For this review, use the dimensioned drawing (mm, ordinates from the lowest corner) and the shaded views. A direction names the side the tool comes from. Give positions to 0.01 mm unless a question says otherwise; leave off trailing zeros. Write each loop counter-clockwise with the first axis right and the second up, starting at its lowest first coordinate (ties: lowest second). Pieces come first, ordered by that corner, then holes. Notation, with made-up numbers: (-13.5, -20) -> (36.5, -20) arc R13 ccw to (36.5, -13) -> close; hole circle Ø3 at (-10.75, 21). An arc over 180 degrees is marked (long way). Answer as CSV lines item,"result".
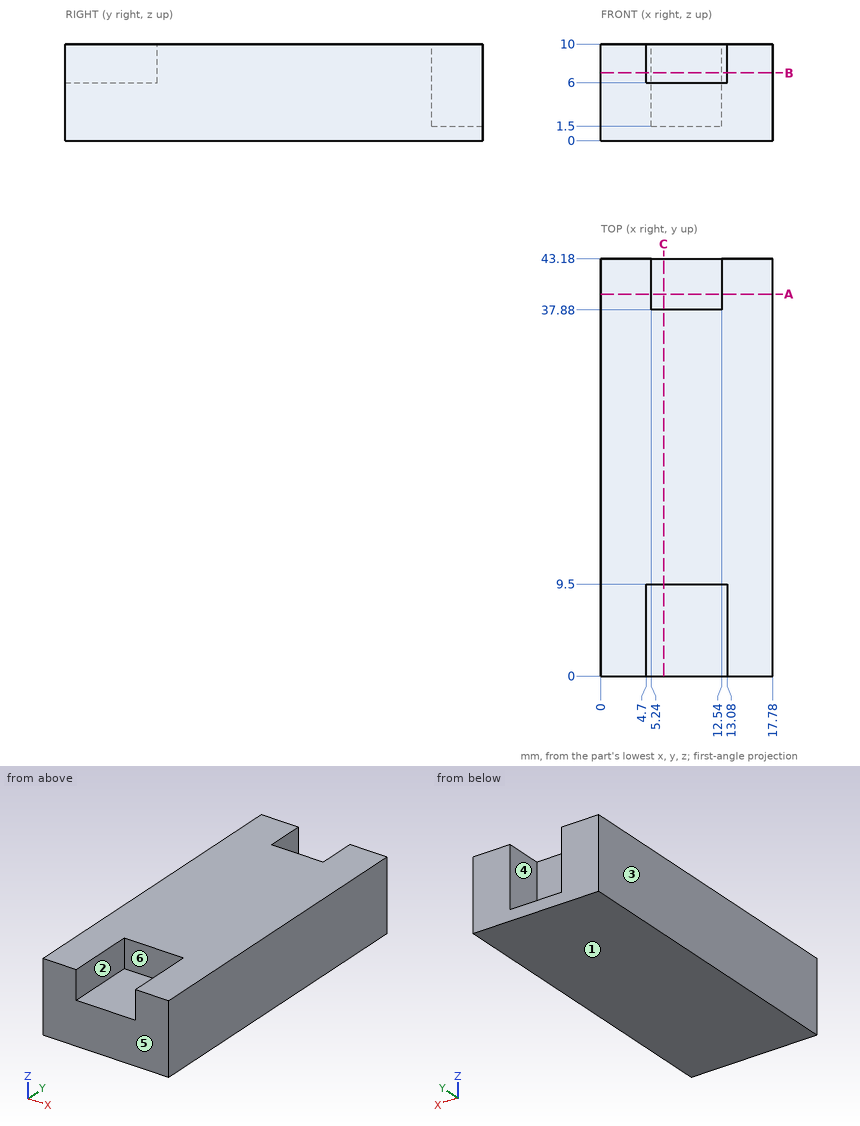
Q1. Add section B-B (z = 7). Write out the cut boundary in (x, y).
Answer block:
outline,"(0, 0) -> (4.7, 0) -> (4.7, 9.5) -> (13.08, 9.5) -> (13.08, 0) -> (17.78, 0) -> (17.78, 43.18) -> (12.54, 43.18) -> (12.54, 37.88) -> (5.24, 37.88) -> (5.24, 43.18) -> (0, 43.18) -> close"
Q2. To check wall thickness, follow probe 1 along Z at (x, y) = (5.75, 7.5); probe 2 along Y at (x, z) = (6.75, 9.25); probe 3 along Y at (x, z) = (7.5, 4.25). State the ranges of each line that lie inside material, in increasing order. Write a range as [from, to].
Answer block:
probe 1,"z = [0, 6]"
probe 2,"y = [9.5, 37.88]"
probe 3,"y = [0, 37.88]"
Q3. Add section A-A (y = 39.5). Write out the cut boundary in (x, z).
Answer block:
outline,"(0, 0) -> (17.78, 0) -> (17.78, 10) -> (12.54, 10) -> (12.54, 1.5) -> (5.24, 1.5) -> (5.24, 10) -> (0, 10) -> close"
Q4. Add section C-C (x = 6.5). Write out the cut boundary in (y, z).
Answer block:
outline,"(0, 0) -> (43.18, 0) -> (43.18, 1.5) -> (37.88, 1.5) -> (37.88, 10) -> (9.5, 10) -> (9.5, 6) -> (0, 6) -> close"
Q5. Draft analysis for pull direction X (two halves, no side actions). For the marked faces 1, 2 and 3, state which applies: released by +X, released by -X, zero draft, split by the parting line, or undercut.
Answer block:
face 1,"zero draft"
face 2,"undercut"
face 3,"released by -X"
Q6. Clearance check with flat-ended pins moving along their axes: pin 1 (4.5 mm diameter, centred on x = 10.5, z = 7.5, fed in from -Y); pin 2 (1 mm diameter, centred on x = 8.5, z = 6, fed in from +Y); pin 3 (2.5 mm diameter, centred on x = 9, y = 41.5, fed in from +Z). State where each tip first meets the part, or that it passes through.
Answer block:
pin 1,"stops at y = 0"
pin 2,"stops at y = 37.88"
pin 3,"stops at z = 1.5"
Q7. For the marked faces 4, 5 and 6, list the 3-axis set-ups (+Z, -Z, +X, -X, +Y, -Y) from which the entire face can be reached by the end or side of a thin tool; tool diameter is ignored.
Answer block:
face 4,"+Z, +Y"
face 5,"+Z, -Z, +X, -X, -Y"
face 6,"+Z, -Y"
